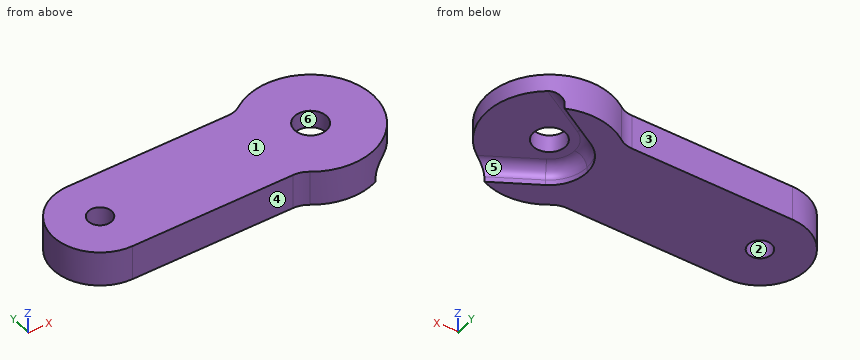
from build123d import *

# Parameters (mm, degrees)
F0_R     = 3.175
F0_R_2   = 4.3434
F1_DEPTH = 9.525
F2_R     = 4.3434
F3_DEPTH = 4.7498
F4_R     = 3.302


with BuildPart() as f1:
    # F0 (on Top) → F1 (new body)
    with BuildSketch(Plane.XY):
        with BuildLine():
            ThreePointArc((-13.577506, -12.7), (-11.642746, -13.001925), (-9.891972, -13.87899))
            ThreePointArc((-9.891972, -13.87899), (17.0434, 0), (-9.891972, 13.87899))
            ThreePointArc((-9.891972, 13.87899), (-11.642746, 13.001925), (-13.577506, 12.7))
            Line((-13.577506, 12.7), (-57.15, 12.7))
            ThreePointArc((-57.15, 12.7), (-69.85, 0), (-57.15, -12.7))
            Line((-57.15, -12.7), (-13.577506, -12.7))
        make_face()
        with Locations((-57.15, 0)):
            Circle(F0_R, mode=Mode.SUBTRACT)
        Circle(F0_R_2, mode=Mode.SUBTRACT)
    extrude(amount=F1_DEPTH)

    # F2 (on face) → F3 (cut)
    with BuildSketch(Plane(origin=(0, 0, 0), x_dir=(1, 0, 0), z_dir=(0, 0, -1))):
        with BuildLine():
            Line((6.770692, 15.640819), (-5.08, 8.798818))
            ThreePointArc((-5.08, 8.798818), (-8.798818, 5.08), (-10.16, 0))
            ThreePointArc((-10.16, 0), (-8.798818, -5.08), (-5.08, -8.798818))
            Line((-5.08, -8.798818), (6.770692, -15.640819))
            ThreePointArc((6.770692, -15.640819), (17.0434, 0), (6.770692, 15.640819))
        make_face()
        Circle(F2_R, mode=Mode.SUBTRACT)
    extrude(amount=-F3_DEPTH, mode=Mode.SUBTRACT)

    # F4
    f4_edges = [f1.edges().sort_by_distance(p)[0] for p in [
        (0.845346, -12.219818, 4.7498),
    ]]
    fillet(f4_edges, radius=F4_R)


solid = f1.part
Read the model definition and answer for the solid it produces. Units are mm, in the model's axes. Face numbers are marked on the shaded views. A direction names the side the tool comes from. Give positions to 0.01 mm unless a question says otherwise; leave off trailing zeros. Write each loop counter-clockwise with the first axis right and the second up, starting at its lowest first coordinate (ties: lowest second). Pieces come first, ordered by that corner, then holes. Notation, with made-up numbers: M -12,70.5 L 1,70.5 A23 cw 1,83.5 Z; hole C -38.75,30 d3. An arc over 180 degrees is marked long. One line per item, written item: value. Start each with the question number.
(1) Find section A-A (x = -15). Determine the outline of the cut face in (y, z) (3 decimals), plus the area to 3 significant figures.
(2) A tool of negligible diameter and unlimited length cuts with its end or side. For the marked faces 4, 5 and 6, from which of +Z, -Z, +X, -X, +Y, -Y can it reach the whole face along a straight path? Write none if from no direction.
(3) Determine the mould class of the marked faces 1, 2 and 3 for opening direction Y: pulls with the +Y half, pulls with the -Y half, needs draft (parallel to the pull), parting line crosses it, or undercut.
(4) Find the intervals of material crossed by line 1 (Y direction, x = 0, z = 6.85); line 2 (X direction, y = -1.5, z = 6); line 3 (Y direction, x = -8, z = 1.25), in increasing order.
(5) Flat-ended cylindrical pins translate along their axes: pin 1 Ø5 at (x, z) = (-38, 2.5) entering from +Y; pin 2 Ø1 at (y, z) = (7, 8) entering from +X; pin 3 Ø1 at (y, z) = (-12, 3) entering from +X; pin 4 Ø4 at (x, y) = (-57.15, 0) entering from +Z. Find the tip coordinate at first contact, or state that the pin passes through.
Results below:
1. outline: M -12.7,0 L 12.7,0 L 12.7,9.525 L -12.7,9.525 Z
1. area: 242 mm^2
2. face 4: +Z, -Z, -X, -Y
2. face 5: -Z, +X
2. face 6: +Z, -Z
3. face 1: needs draft
3. face 2: undercut
3. face 3: pulls with the +Y half
4. line 1: y = -17.04 to -4.34, 4.34 to 17.04
4. line 2: x = -69.76 to -59.95, -54.35 to -4.08, 4.08 to 16.98
4. line 3: y = -15.05 to -6.26, 6.26 to 15.05
5. pin 1: stops at y = 12.7
5. pin 2: stops at x = 15.76
5. pin 3: stops at x = 2.29
5. pin 4: passes through
